Read the model definition and answer for the solid it produces. Units are mm, in the model's axes. Face numbers are marked on the shaded views. Give positions to 0.01 mm unless a question says otherwise; leave off trailing zeros. Order: outer loops, then holes, each group sorted by start corner. A loop starts at its lowest first (then second) coordinate and runs counter-clockwise, first axis right, second up. Notation, with made-up numbers: (-32.75, 62.5) - (-17.75, 62.5) arc R26 ccw to (-17.75, 86.5) - close; hole circle Ø10 at (-20, 34). An arc over 180 degrees is marked (long way). Write item = value, one per line.
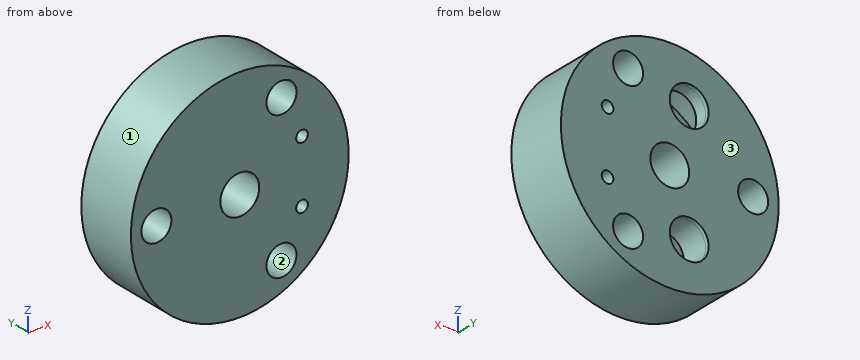
Autodesk Inventor part; units mm, degrees
ref_plane "YZ Plane" through (0, 0, 0) normal (1, 0, 0) x (0, 1, 0)
ref_plane "XZ Plane" through (0, 0, 0) normal (0, 1, 0) x (-1, 0, 0)
ref_plane "XY Plane" through (0, 0, 0) normal (0, 0, 1) x (1, 0, 0)
sketch "Sketch1" plane through (0, 0, 0) normal (0, 1, 0) x (-1, 0, 0)
  circle A0 centre (0, 0) radius 17.78
  dimension "d0" = 35.56
extrude "Extrusion1" add sketch "Sketch1" along normal blind 10.16
sketch "Sketch2" plane through (0, 10.16, 0) normal (0, 1, 0) x (1, 0, 0)
  circle A0 centre (0, 0) radius 17.78
hole "Hole1" at (0, 10.16, 0) direction (0, -1, 0) diameter 6.35 end through all
sketch "Sketch3" plane through (0, 10.16, 0) normal (0, 1, 0) x (1, 0, 0)
  line L0 (0, 0) -> (-13.6144, 0)
  dimension "d10" = 13.6144
hole "Hole2" at (-13.6144, 10.16, 0) direction (0, -1, 0) diameter 4.9022 end through all
pattern_circular "Circular Pattern1" count 3 over 360 about axis through (0, -41.1455, 0) along (0, 1, 0) of "Hole2"
sketch "Sketch23" plane through (0, 10.16, 0) normal (0, 1, 0) x (1, 0, 0)
  line L0 (0, 0) -> (10.16, 0)
  line L1 (10.16, 0) -> (10.16, 5.08)
  line L2 (10.16, 5.08) -> (10.16, -5.08)
  dimension "d122" = 10.16
  dimension "d123" = 5.08
  dimension "d124" = 10.16
hole "Hole10" at (10.16, 10.16, -5.08) at (10.16, 10.16, 5.08) direction (0, -1, 0) diameter 1.905 end through all
shell "Shell4" thickness 0.635 removed faces 0
sketch "Sketch26" plane through (0, 10.16, 0) normal (0, 1, 0) x (1, 0, 0)
  line L0 (0, 0) -> (-3.175, 9.6512)
  line L1 (-3.175, 9.6512) -> (0, 0)
  line L2 (0, 0) -> (-3.175, -9.6512)
  dimension "d148" = 10.16
  dimension "d149" = 10.16
hole "Hole12" at (-3.175, 10.16, -9.6512) at (-3.175, 10.16, 9.6512) direction (0, -1, 0) diameter 6.35 depth 2.54
sketch "Sketch27" plane through (0, 10.16, 0) normal (0, 1, 0) x (1, 0, 0)
  circle A0 centre (-3.175, 9.6512) radius 3.175
  circle A1 centre (-3.175, 9.6512) radius 3.81
  circle A2 centre (-3.175, -9.6512) radius 3.175
  circle A3 centre (-3.175, -9.6512) radius 3.81
  point P0 (0, 0)
  dimension "d157" = 7.62
  dimension "d158" = 7.62
extrude "Extrusion15" add sketch "Sketch27" against normal blind 5.08 contours A1
extrude "Extrusion16" add sketch "Sketch27" against normal blind 2.54 contours A3
sketch "Sketch28" plane through (0, 10.16, 0) normal (0, 1, 0) x (1, 0, 0)
  point P0 (0, 0)
properties part number "water"
1. Section C-C (z = -5.08) is taken. Determine the outline of the cut face in (x, y) (1 decimal).
Recorded:
outline = (-17, 0) - (9.2, 0) - (9.2, 10.2) - (-17, 10.2) - close; (11.1, 0) - (17, 0) - (17, 10.2) - (11.1, 10.2) - close; hole (-16.4, 0.6) - (8.6, 0.6) - (8.6, 9.5) - (-16.4, 9.5) - close; hole (11.7, 0.6) - (16.4, 0.6) - (16.4, 9.5) - (11.7, 9.5) - close
2. Determine the mould class of the marked faces 1, 2 and 3 for opening direction Z: +Z half, -Z half, draft (parallel to the pull), parting line (faces both ways), or undercut.
Recorded:
face_1 = parting line
face_2 = undercut
face_3 = draft
3. Section D-D (y = 2.5) is taken. Count the separate pieces of the cut face and the enclosed holes in it, and give its area (3 significant figures).
Recorded:
separate_pieces = 7
enclosed_holes = 7
area = 127 mm^2
4. Straight lines are drawn through the part: L1, parallel to Y at x = 11, z = 10 (3 decimals); L2, parallel to X at y = 6.75, z = -11.5; L3, parallel to X at y = 3.5, z = 12. For each, find the intervals that lie inside material, in ascending order. Write a range as [from, to].
Recorded:
L1 = [0, 0.635], [9.525, 10.16]
L2 = [-13.56, -12.72], [-6.51, -5.76], [-0.59, 0.16], [3.73, 4.37], [9.24, 9.88], [12.72, 13.56]
L3 = [-13.12, -12.25], [3.73, 4.37], [9.25, 9.89], [12.25, 13.12]
5. Section A-A (z = 0) is taken. Determine the outline of the cut face in (x, y) (1 decimal), and give its area (3 significant figures).
Recorded:
outline = (-17.8, 0) - (-16.1, 0) - (-16.1, 10.2) - (-17.8, 10.2) - close; (-11.2, 0) - (-3.2, 0) - (-3.2, 10.2) - (-11.2, 10.2) - close; (3.2, 0) - (17.8, 0) - (17.8, 10.2) - (3.2, 10.2) - close; hole (-17.1, 0.6) - (-16.7, 0.6) - (-16.7, 9.5) - (-17.1, 9.5) - close; hole (-10.5, 0.6) - (-3.8, 0.6) - (-3.8, 9.5) - (-10.5, 9.5) - close; hole (3.8, 0.6) - (17.1, 0.6) - (17.1, 9.5) - (3.8, 9.5) - close
area = 64.7 mm^2
6. Section B-B (x = -15) is taken. Determine the outline of the cut face in (y, z) (3 decimals).
Recorded:
outline = (0, -9.546) - (10.16, -9.546) - (10.16, -2.022) - (0, -2.022) - close; (0, 2.022) - (10.16, 2.022) - (10.16, 9.546) - (0, 9.546) - close; hole (0.635, -8.304) - (9.525, -8.304) - (9.525, -2.758) - (0.635, -2.758) - close; hole (0.635, 2.758) - (9.525, 2.758) - (9.525, 8.304) - (0.635, 8.304) - close
7. Flat-ended cylindrical pins translate along their axes: pin 1 (5 mm diameter, centred on x = -11, y = 1.5, fed in from -Z); pin 2 (4 mm diameter, centred on x = 0, z = 0, fed in from -Y); pin 3 (1 mm diameter, centred on y = 6.5, z = -14, fed in from +X); pin 4 (1.5 mm diameter, centred on x = -5, y = 9, fed in from +Z). Find the tip coordinate at first contact, or state that the pin passes through.
Recorded:
pin_1 = -15.62
pin_2 = through
pin_3 = 11.57
pin_4 = 17.26
